Part model, mm, in its own coordinate system. A direction names the side the tool comes from. Give positions to 0.01 mm unless a question says otherwise; leave off trailing zeros. Write each loop counter-clockwise with the first axis right and the second up, starting at its lowest first coordinate (ties: lowest second). Pieces come first, ordered by that corner, then holes. Notation, with made-up numbers: M 24.25,47 L 61.25,47 A26 cw 61.25,78 Z; hole C 40,-10.5 d6. An arc over 180 degrees is marked long. Use a Markdown table: item, result. Add a question column.
from build123d import *

# Parameters (mm, degrees)
F0_R     = 50
F1_DEPTH = 10.668
F2_R     = 9.525
F3_DEPTH = 6.35
F4_R     = 1.905
F5_DEPTH = 25.4
F6_R     = 5
F7_DEPTH = 101.6


with BuildPart() as f1:
    # F0 (on Top) → F1 (new body)
    with BuildSketch(Plane.XY):
        Circle(F0_R)
    extrude(amount=F1_DEPTH)

    # F2 (on face) → F3 (join)
    with BuildSketch(Plane.XY.offset(10.668)):
        Circle(F2_R)
    extrude(amount=F3_DEPTH)

    # F4 (on Right) → F5 (cut)
    with BuildSketch(Plane.YZ):
        with Locations((0, 13.843)):
            Circle(F4_R)
    extrude(amount=-F5_DEPTH, mode=Mode.SUBTRACT)

    # F6 (on face) → F7 (cut)
    with BuildSketch(Plane(origin=(0, 0, 0), x_dir=(1, 0, 0), z_dir=(0, 0, -1))):
        Circle(F6_R)
    extrude(amount=-F7_DEPTH, mode=Mode.SUBTRACT)

    # F8 (on Right) → F9 (revolve, cut)
    with BuildSketch(Plane.YZ):
        with BuildLine():
            Line((-50.066398, 8.67579), (-50.066398, 7.502463))
            ThreePointArc((-50.066398, 7.502463), (-51.774357, 5.118554), (-50.042302, 2.752094))
            Line((-50.042302, 2.752094), (-50.042302, 1.583694))
            Line((-50.042302, 1.583694), (-41.154411, 2.780473))
            Line((-41.154411, 2.780473), (-41.154411, 7.307734))
            Line((-41.154411, 7.307734), (-50.066398, 8.67579))
        make_face()
    revolve(axis=Axis((0, 0, 17.018), (0, 0, 1)), mode=Mode.SUBTRACT)


solid = f1.part
1. Drill centre lines: probe 1 along Z at (x, y) = (-8.25, 0); probe 2 along Z at (x, y) = (-36.5, 18.5); probe 3 along Z at (x, y) = (7.5, 45.5). Where is each one in solid material? Low to high. Write a range as [from, to].
2. Flat gauge pins, fed straight in: pin 1 (1.5 mm diameter, centred on y = 15, z = 8, fed in from -X); pin 2 (6 mm diameter, centred on y = 0, z = 13.843, fed in from -X) (3 decimals); pin 3 (1 mm diameter, centred on x = 0.5, z = 6, fed in from +Y). Where does each tip first touch, or does it go through?
3. Mould opens along Z. For faces 5 (the conical face through (-40.716, 9.041, 7.393)), 6 (the flat face through (-1, -10, 0)), 7 (the flat face through (4, -4, 17.018)) say: released by +Z, released by -Z, zero draft, split by the parting line, or undercut.
4. Cut at B-B (x = 0). Write the cut outline in (y, z) (3 decimals).
5. Cut at A-A (y = 0). Write the cut outline in (x, z) (3 decimals), then the cut area to 3 significant figures.
6. Tool access for faces 1 (the cylindrical face through (47.69, 15.02, 0.78)), 2 (the cylindrical face through (9.085, 2.861, 13.799)), 3 (the conical face through (-25.303, 33, 2.723)), 4 (the cylindrical face through (-7.042, -1.903, 13.927)): list every direction of +Z, -Z, +X, -X, +Y, -Y with a clear straight run to the whole face (end or side of a thin tool).
A:
| question | item | result |
|---|---|---|
| 1 | probe 1 | z = [0, 11.94], [15.75, 17.02] |
| 1 | probe 2 | z = [0, 10.67] |
| 1 | probe 3 | z = [0, 2.11], [8.07, 10.67] |
| 2 | pin 1 | stops at x = -47.8 |
| 2 | pin 2 | stops at x = -9.525 |
| 2 | pin 3 | stops at y = 41.15 |
| 3 | face 5 | undercut |
| 3 | face 6 | released by -Z |
| 3 | face 7 | released by +Z |
| 4 | outline | M -50,0 L -5,0 L -5,17.018 L -9.525,17.018 L -9.525,10.668 L -50,10.668 L -50,8.666 L -41.154,7.308 L -41.154,2.78 L -50,1.589 Z; M 5,0 L 50,0 L 50,1.589 L 41.154,2.78 L 41.154,7.308 L 50,8.666 L 50,10.668 L 9.525,10.668 L 9.525,17.018 L 5,17.018 Z |
| 5 | outline | M -50,0 L -5,0 L -5,11.938 L -9.525,11.938 L -9.525,10.668 L -50,10.668 L -50,8.666 L -41.154,7.308 L -41.154,2.78 L -50,1.589 Z; M -9.525,15.748 L -5,15.748 L -5,17.018 L -9.525,17.018 Z; M 5,0 L 50,0 L 50,1.589 L 41.154,2.78 L 41.154,7.308 L 50,8.666 L 50,10.668 L 9.525,10.668 L 9.525,17.018 L 5,17.018 Z |
| 5 | area | 898 mm² |
| 6 | face 1 | +Z, -Z |
| 6 | face 2 | +Z |
| 6 | face 3 | none |
| 6 | face 4 | -X |
